Design review of the part built by this model. Coordinates are the model's own, in mm. A direction names the side the tool comes from. Coordinates: 2 decimals unless noted, no trailing zeros. Order: outer loops, then holes, each group sorted by start corner. A loop starts at its lowest first (then second) coordinate and runs counter-clockwise, first axis right, second up. Notation, with made-up numbers: M 42.25,31.5 L 84.25,31.5 A37 ccw 84.25,70.5 Z; hole C 84,84.5 d8. An arc over 180 degrees is marked long. Answer as a JSON object with one key per item and string values.
from build123d import *

# Parameters (mm, degrees)
BOSS_EXTRUDE1_DEPTH = 2.5
SKETCH2_R           = 0.9
CUT_EXTRUDE1_DEPTH  = 2.5
SKETCH3_W           = 14.34
SKETCH3_H           = 9.878404361
BOSS_EXTRUDE2_DEPTH = 4.5
SKETCH4_R           = 3.05
CUT_EXTRUDE2_DEPTH  = 57.133646482
SKETCH5_W           = 6.098404361
SKETCH5_H           = 2.9
CUT_EXTRUDE3_DEPTH  = 57.133646482
FILLET1_R           = 4
SKETCH7_W           = 6.34
SKETCH7_H           = 3.5
CUT_EXTRUDE5_DEPTH  = 61.145372561
FILLET2_R           = 1


with BuildPart() as part:
    # Sketch1 → Boss-Extrude1 (new body)
    with BuildSketch(Plane(origin=(0, 0, 0), x_dir=(1, 0, 0), z_dir=(0, 1, 0))):
        Polygon((26.473858297, -52.017754202), (24.673858297, -53.817754202), (13.933858297, -53.817754202), (12.133858297, -52.017754202), (12.133858297, -38.739349841), (13.933858297, -36.939349841), (24.673858297, -36.939349841), (26.473858297, -38.739349841), align=None)
    extrude(amount=BOSS_EXTRUDE1_DEPTH)

    # Sketch2 → Cut-Extrude1 (cut)
    with BuildSketch(Plane(origin=(0, 2.5, 0), x_dir=(1, 0, 0), z_dir=(0, 1, 0))):
        with Locations(Location((24.303858297, -52.377754202, 0), (0, 0, 270))):
            Circle(SKETCH2_R)
        with Locations(Location((14.303858297, -52.377754202, 0), (0, 0, 270))):
            Circle(SKETCH2_R)
        with Locations(Location((14.303858297, -38.379349841, 0), (0, 0, 270))):
            Circle(SKETCH2_R)
        with Locations(Location((24.303858297, -38.379349841, 0), (0, 0, 270))):
            Circle(SKETCH2_R)
    extrude(amount=-CUT_EXTRUDE1_DEPTH, mode=Mode.SUBTRACT)

    # Sketch3 → Boss-Extrude2 (add)
    with BuildSketch(Plane(origin=(0, 2.5, 0), x_dir=(1, 0, 0), z_dir=(0, 1, 0))):
        with Locations((19.303858297, -45.378552021)):
            Rectangle(SKETCH3_W, SKETCH3_H)
    extrude(amount=BOSS_EXTRUDE2_DEPTH)

    # Sketch4 → Cut-Extrude2 (cut, through all)
    with BuildSketch(Plane.ZY.offset(-12.133858297)):
        with Locations((45.377754202, 2.9)):
            Circle(SKETCH4_R)
    extrude(amount=-CUT_EXTRUDE2_DEPTH, mode=Mode.SUBTRACT)

    # Sketch5 → Cut-Extrude3 (cut, through all)
    with BuildSketch(Plane.ZY.offset(-12.133858297)):
        with Locations((45.378552021, 1.45)):
            Rectangle(SKETCH5_W, SKETCH5_H)
    extrude(amount=-CUT_EXTRUDE3_DEPTH, mode=Mode.SUBTRACT)

    # Fillet1
    fillet1_edges = [part.edges().sort_by_distance(p)[0] for p in [
        (19.303858297, 7, 40.439349841),
        (19.303858297, 7, 50.317754202),
    ]]
    fillet(fillet1_edges, radius=FILLET1_R)

    # Sketch7 → Cut-Extrude5 (cut, through all)
    with BuildSketch(Plane(origin=(0, 2.5, 0), x_dir=(1, 0, 0), z_dir=(0, 1, 0))):
        with Locations((19.303858297, -52.067754202)):
            Rectangle(SKETCH7_W, SKETCH7_H)
        with Locations((19.303858297, -38.689349841)):
            Rectangle(SKETCH7_W, SKETCH7_H)
    extrude(amount=-CUT_EXTRUDE5_DEPTH, mode=Mode.SUBTRACT)

    # Fillet2
    fillet2_edges = [part.edges().sort_by_distance(p)[0] for p in [
        (22.473858297, 1.25, 50.317754202),
        (22.473858297, 1.25, 53.817754202),
        (16.133858297, 1.25, 53.817754202),
        (16.133858297, 1.25, 50.317754202),
        (22.473858297, 1.25, 36.939349841),
        (22.473858297, 1.25, 40.439349841),
        (16.133858297, 1.25, 40.439349841),
        (16.133858297, 1.25, 36.939349841),
    ]]
    fillet(fillet2_edges, radius=FILLET2_R)


solid = part.part
1) Add section B-B (y = 3.75). State the section outline as (x, z) points, and give its area (3 significant figures).
Taken from the geometry:
{"outline": "M 12.13,40.51 L 26.47,40.51 L 26.47,42.45 L 12.13,42.45 Z; M 12.13,48.31 L 26.47,48.31 L 26.47,50.25 L 12.13,50.25 Z", "area": "55.6 mm2"}
2) Tool access review of faces 4 (the flat face through (14, 2.5, 51)), 5 (the cylindrical face through (16.43, 1.23, 40.15)), 6 (the cylindrical face through (22.17, 1.23, 50.6)): name each direction out of +Z, -Z, +X, -X, +Y, -Y from which nothing blocks a thin tool from reaching the whole face with its end or side.
Taken from the geometry:
{"face 4": "+Z, +X, -X, +Y", "face 5": "-Z, +Y, -Y", "face 6": "+Z, +Y, -Y"}
3) To check wall thickness, follow L1, parallel to Z at x = 20, y = 3.25; L2, parallel to Z at x = 15, y = 5; L3, parallel to Y at x = 14.75, z = 45.5. State the ranges of each line that lie inside material, in increasing order.
Taken from the geometry:
{"L1": "z = 40.45 to 42.35, 48.41 to 50.31", "L2": "z = 40.98 to 43.17, 47.59 to 49.78", "L3": "y = 5.95 to 7"}
4) Mouldability with a two-part tool opening along Z and no side actions: class faces 1 (the flat face through (19, 0, 50)), 2 (the cylindrical face through (25.2, 1.3, 38.3)), 3 (the cylindrical face through (19.4, 5.86, 41.64)) as released by +Z, released by -Z, zero draft, split by the parting line, or undercut.
Taken from the geometry:
{"face 1": "zero draft", "face 2": "undercut", "face 3": "released by -Z"}
5) Add section C-C (x = 18.5). State the section outline as (y, z) points.
Taken from the geometry:
{"outline": "M 0,40.44 L 3,40.44 A4 ccw 7,44.44 L 7,46.32 A4 ccw 3,50.32 L 0,50.32 L 0,48.43 L 2.9,48.43 A3.05 cw long 2.8,42.33 L 0,42.33 Z"}
6) Add section A-A (z = 39). State the section outline as (x, y) points.
Taken from the geometry:
{"outline": "M 12.13,0 L 13.65,0 L 13.65,2.5 L 12.13,2.5 Z; M 14.96,0 L 16.13,0 L 16.13,2.5 L 14.96,2.5 Z; M 22.47,0 L 23.65,0 L 23.65,2.5 L 22.47,2.5 Z; M 24.96,0 L 26.47,0 L 26.47,2.5 L 24.96,2.5 Z"}
7) Add section D-D (y = 4.75). State the section outline as (x, z) points, and give its area (3 significant figures).
Taken from the geometry:
{"outline": "M 12.13,40.84 L 26.47,40.84 L 26.47,42.95 L 12.13,42.95 Z; M 12.13,47.8 L 26.47,47.8 L 26.47,49.91 L 12.13,49.91 Z", "area": "60.5 mm2"}
8) Insertion check: pin 1 Ø1.5 at (x, y) = (20.5, 6) entering from -Z; pin 2 Ø3.5 at (x, y) = (22.5, 1) entering from +Z; pin 3 Ø1 at (x, y) = (20.5, 5.5) entering from +Z; pin 4 Ø3 at (x, z) = (25, 51.5) entering from +Y. Each pin has a flat end and moves straight along its axis. Give the tip position at first contact, or say it passes through.
Taken from the geometry:
{"pin 1": "stops at z = 41.13", "pin 2": "stops at z = 53.82", "pin 3": "stops at z = 49.78", "pin 4": "stops at y = 4.56"}
